Design review of the part built by this model. Coordinates are the model's own, in mm. Face numbers are marked on the shaded views. A direction names the side the tool comes from. Round coordinates to 2 decimals unless told otherwise and drop trailing zeros. Write each loop counter-clockwise with the first axis right and the second up, starting at its lowest first coordinate (ties: lowest second). Pieces come first, ordered by that corner, then holes. Notation, with made-up numbers: M 79,84 L 103,84 A23 ccw 103,120 Z; hole C 5,-9.75 d1. An arc over 180 degrees is marked long. One line per question, with ' | ' between items. Start each with the question number.
Item 1: Add section A-A, the plane z = 90. State the section outline as (x, y) points.
Item 2: Add section D-D, the plane z = 39.5. State the section outline as (x, y) points.
Item 3: Machinability: for the marked faces 1 and 2, which of the approach directions +Z, -Z, +X, -X, +Y, -Y give a long, thin tool a straight path to every point of the face, cutting with its end or side? Answer none if there is none.
Item 4: Insertion check: pin 1 Ø5 at (x, z) = (29.5, 70.5) entering from -Y. The pin has a flat end and moves straight along its axis. Give the tip position at first contact, or say it passes through.
Item 5: For L1, parallel to X at y = -31.5, z = 85.5; L2, parallel to Z at x = -19.5, y = 113; L3, parallel to Y at x = 36.5, z = 103, list the stretches that pass through material, from the lowest coordinate up.
Item 6: Add section B-B, the plane y = 124.5. State the section outline as (x, z) points, and give its area (3 significant figures).
Item 7: Draft analysis for pull direction X (two halves, no side actions). For the marked faces 3, 4 and 5, state which applies: released by +X, released by -X, zero draft, split by the parting line, or undercut.
Item 8: Add section C-C, the plane x = -154. State the section outline as (y, z) points.
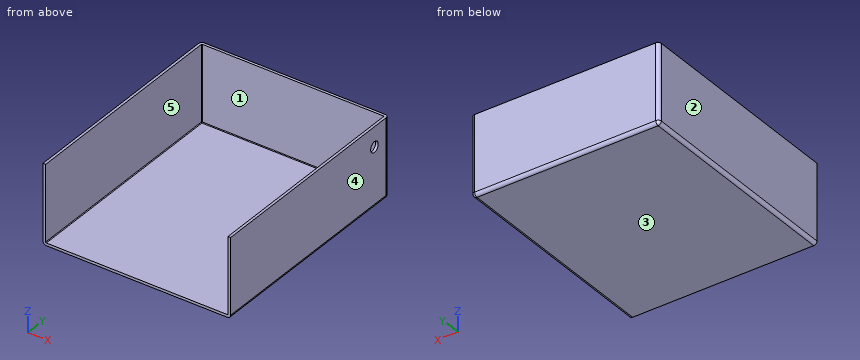
```python
from build123d import *

# Parameters (mm, degrees)
F0_W     = 285
F0_H     = 335
F1_DEPTH = 120
F2_R     = 5
F3_T     = -4
F5_D     = 16
F5_DEPTH = 10


with BuildPart() as f1:
    # F0 (on Top) → F1 (new body)
    with BuildSketch(Plane.XY):
        with Locations((-80.726171, 114.31913)):
            Rectangle(F0_W, F0_H)
    extrude(amount=F1_DEPTH)

    # F2
    f2_edges = [f1.edges().sort_by_distance(p)[0] for p in [
        (-223.226171, 114.31913, 0),
        (-80.726171, 281.81913, 0),
        (61.773829, 114.31913, 0),
        (-223.226171, 281.81913, 60),
        (61.773829, 281.81913, 60),
    ]]
    fillet(f2_edges, radius=F2_R)

    # F3
    f3_openings = [f1.faces().sort_by_distance(p)[0] for p in [
        (-80.726171, 114.300429, 120),
        (-80.726171, -53.18087, 60.01848),
    ]]
    offset(amount=F3_T, openings=f3_openings)

    # F5
    with Locations(Plane.YZ.offset(61.773829)):
        with Locations((251.81913, 90)):
            Hole(F5_D / 2, depth=F5_DEPTH)


solid = f1.part
```
Computed values:
1) outline: M -223.23,-53.18 L -219.23,-53.18 L -219.23,276.82 A1 cw -218.23,277.82 L 56.77,277.82 A1 cw 57.77,276.82 L 57.77,259.82 L 61.77,259.82 L 61.77,276.82 A5 ccw 56.77,281.82 L -218.23,281.82 A5 ccw -223.23,276.82 Z; M 57.77,-53.18 L 61.77,-53.18 L 61.77,243.82 L 57.77,243.82 Z
2) outline: M -223.23,-53.18 L -219.23,-53.18 L -219.23,276.82 A1 cw -218.23,277.82 L 56.77,277.82 A1 cw 57.77,276.82 L 57.77,-53.18 L 61.77,-53.18 L 61.77,276.82 A5 ccw 56.77,281.82 L -218.23,281.82 A5 ccw -223.23,276.82 Z
3) face 1: +Z, -Y | face 2: +Z, -Z, -X, +Y, -Y
4) pin 1: stops at y = 277.82
5) L1: x = -223.23 to -219.23, 57.77 to 61.77 | L2: z = 0 to 4 | L3: y = 277.82 to 281.82
6) outline: M -223.23,5 A5 ccw -218.23,0 L 56.77,0 A5 ccw 61.77,5 L 61.77,120 L 57.77,120 L 57.77,5 A1 cw 56.77,4 L -218.23,4 A1 cw -219.23,5 L -219.23,120 L -223.23,120 Z | area: 2,060 mm^2
7) face 3: zero draft | face 4: released by +X | face 5: undercut
8) outline: M -53.18,0 L 276.82,0 A5 ccw 281.82,5 L 281.82,120 L 277.82,120 L 277.82,5 A1 cw 276.82,4 L -53.18,4 Z
